Source: three-view drawing plus pictorial views. Frame: mm from the lowest corner of the part. A direction names the side the tool comes from. Coordinates: 2 decimals unless noted, no trailing zeros. Loops run counter-clockwise (first coordinate to the right, second up) from the corner with the lowest first, then second, coordinate; pieces in that order, holes last. Notation, with made-up numbers: (70.25, 16.5) - (112.25, 16.5) arc R21 cw to (112.25, 21.5) - close; hole circle Ø5 at (-31, 9). An arc over 180 degrees is marked (long way). Return JSON: item names as keys, results as strings.
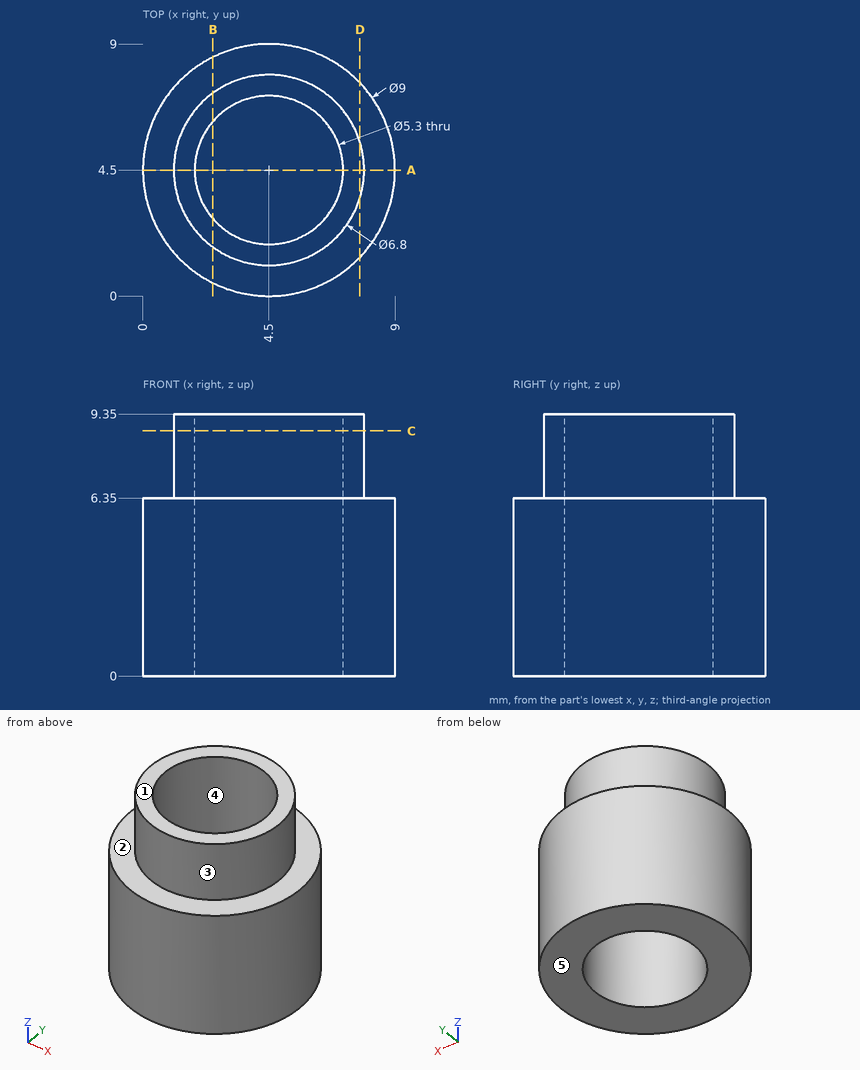
Item 1: Section query D-D, the plane x = 7.75. Return loops of the section in (y, z).
Worked out:
{"outline": "(1.39, 0) - (7.61, 0) - (7.61, 6.35) - (5.5, 6.35) - (5.5, 9.35) - (3.5, 9.35) - (3.5, 6.35) - (1.39, 6.35) - close"}
Item 2: Section query C-C, the plane z = 8.75. Return loops of the section in (x, y).
Worked out:
{"outline": "circle Ø6.8 at (4.5, 4.5); hole circle Ø5.3 at (4.5, 4.5)"}
Item 3: Section query B-B, the plane x = 2.5. Return loops of the section in (y, z).
Worked out:
{"outline": "(0.47, 0) - (2.76, 0) - (2.76, 9.35) - (1.75, 9.35) - (1.75, 6.35) - (0.47, 6.35) - close; (6.24, 0) - (8.53, 0) - (8.53, 6.35) - (7.25, 6.35) - (7.25, 9.35) - (6.24, 9.35) - close"}
Item 4: Reachability of the marked faces 1 and 2 from +Z, -Z, +X, -X, +Y, -Y: full face, straight path, thin tool, end or side. Return the list, or none.
Worked out:
{"face 1": "+Z, +X, -X, +Y, -Y", "face 2": "+Z"}
Item 5: Ray query, probe 1 along Y at (x, z) = (4.5, 7); probe 2 along Y at (x, z) = (4.5, 4); probe 3 along Z at (x, y) = (0.5, 3.75). Return the intervals inside material, ascending. Write a range as from..to.
Worked out:
{"probe 1": "1.1..1.85, 7.15..7.9", "probe 2": "0..1.85, 7.15..9", "probe 3": "0..6.35"}
Item 6: First-contact query: pin 1 Ø1 at (x, y) = (3.5, 5) entering from -Z; pin 2 Ø1 at (x, z) = (7.5, 8) entering from -Y; pin 3 Ø1.5 at (x, y) = (6, 1) entering from +Z. Flat tips, straight axial feed; report the tip coordinate or a pass-through.
Worked out:
{"pin 1": "through", "pin 2": "y = 2.2", "pin 3": "z = 9.35"}
Item 7: Mould query, pull axis Y, two halves, no side actions, for the marked faces 3, 4 and 5. Classes: +Y half, -Y half, draft (parallel to the pull), parting line (faces both ways), or undercut.
Worked out:
{"face 3": "parting line", "face 4": "undercut", "face 5": "draft"}
Item 8: Section query A-A, the plane y = 4.5. Return loops of the section in (x, z).
Worked out:
{"outline": "(0, 0) - (1.85, 0) - (1.85, 9.35) - (1.1, 9.35) - (1.1, 6.35) - (0, 6.35) - close; (7.15, 0) - (9, 0) - (9, 6.35) - (7.9, 6.35) - (7.9, 9.35) - (7.15, 9.35) - close"}
